from build123d import *

# Parameters (mm, degrees)
SKETCH1_W           = 151
SKETCH1_H           = 101.6
BOSS_EXTRUDE1_DEPTH = 3.8
SKETCH3_W           = 1.5
SKETCH3_H           = 3.5
CUT_EXTRUDE1_DEPTH  = 183.038457475
SKETCH4_W           = 10
SKETCH4_H           = 101.6
BOSS_EXTRUDE2_DEPTH = 3.8
SKETCH5_R           = 3
SKETCH5_R_2         = 1.75
CUT_EXTRUDE2_DEPTH  = 191.415335517
FILLET1_R           = 3
FILLET2_R           = 3
SKETCH6_W           = 3.8
SKETCH6_H           = 5.8
SKETCH6_H_2         = 10
SKETCH6_W_2         = 10
SKETCH6_H_3         = 3.8
SKETCH6_H_4         = 5
CUT_EXTRUDE3_DEPTH  = 191.415335517


with BuildPart() as part:
    # Sketch1 → Boss-Extrude1 (new body)
    with BuildSketch(Plane(origin=(0, 0, 0), x_dir=(1, 0, 0), z_dir=(0, 1, 0))):
        with Locations((75.5, -50.8)):
            Rectangle(SKETCH1_W, SKETCH1_H)
    extrude(amount=BOSS_EXTRUDE1_DEPTH)

    # Sketch3 → Cut-Extrude1 (cut, through all)
    with BuildSketch(Plane.XZ):
        with Locations((40.75, 87.6)):
            Rectangle(SKETCH3_W, SKETCH3_H)
        with Locations((48.25, 87.6)):
            Rectangle(SKETCH3_W, SKETCH3_H)
        with Locations((134.25, 87.6)):
            Rectangle(SKETCH3_W, SKETCH3_H)
        with Locations((141.75, 87.6)):
            Rectangle(SKETCH3_W, SKETCH3_H)
    extrude(amount=-CUT_EXTRUDE1_DEPTH, mode=Mode.SUBTRACT)

    # Sketch4 → Boss-Extrude2 (add, through all)
    with BuildSketch(Plane.XZ):
        with Locations((156, 50.8)):
            Rectangle(SKETCH4_W, SKETCH4_H)
    extrude(amount=-BOSS_EXTRUDE2_DEPTH)

    # Sketch5 → Cut-Extrude2 (cut, through all)
    with BuildSketch(Plane.XZ):
        with Locations(Location((155, 50.8, 0), (0, 0, 270))):
            Circle(SKETCH5_R)
        with Locations(Location((155, 91.6, 0), (0, 0, 270))):
            Circle(SKETCH5_R_2)
        with Locations(Location((155, 10, 0), (0, 0, 270))):
            Circle(SKETCH5_R_2)
    extrude(amount=-CUT_EXTRUDE2_DEPTH, mode=Mode.SUBTRACT)

    # Fillet1
    fillet1_edges = [part.edges().sort_by_distance(p)[0] for p in [
        (0, 1.9, 0),
        (0, 1.9, 101.6),
    ]]
    fillet(fillet1_edges, radius=FILLET1_R)

    # Fillet2
    fillet2_edges = [part.edges().sort_by_distance(p)[0] for p in [
        (161, 1.9, 101.6),
        (161, 1.9, 0),
    ]]
    fillet(fillet2_edges, radius=FILLET2_R)

    # Sketch6 → Cut-Extrude3 (cut, through all)
    with BuildSketch(Plane(origin=(0, 3.8, 0), x_dir=(1, 0, 0), z_dir=(0, 1, 0))):
        Polygon((148, -94), (148, -89.8), (144.2, -89.8), (144.2, -94.8), (138, -94.8), (138, -98.6), (148, -98.6), align=None)
        with Locations((146.1, -78.1)):
            Rectangle(SKETCH6_W, SKETCH6_H)
        with Locations((146.1, -51.8)):
            Rectangle(SKETCH6_W, SKETCH6_H_2)
        with Locations((146.1, -31.8)):
            Rectangle(SKETCH6_W, SKETCH6_H_2)
        with Locations((146.1, -11.8)):
            Rectangle(SKETCH6_W, SKETCH6_H_2)
        with Locations((135.5, -4.9)):
            Rectangle(SKETCH6_W_2, SKETCH6_H_3)
        with Locations((115.5, -4.9)):
            Rectangle(SKETCH6_W_2, SKETCH6_H_3)
        with Locations((95.5, -4.9)):
            Rectangle(SKETCH6_W_2, SKETCH6_H_3)
        with Locations((75.5, -4.9)):
            Rectangle(SKETCH6_W_2, SKETCH6_H_3)
        with Locations((55.5, -4.9)):
            Rectangle(SKETCH6_W_2, SKETCH6_H_3)
        with Locations((35.5, -4.9)):
            Rectangle(SKETCH6_W_2, SKETCH6_H_3)
        with Locations((15.5, -4.9)):
            Rectangle(SKETCH6_W_2, SKETCH6_H_3)
        with Locations((4.9, -11.8)):
            Rectangle(SKETCH6_W, SKETCH6_H_2)
        with Locations((4.9, -31.8)):
            Rectangle(SKETCH6_W, SKETCH6_H_2)
        with Locations((4.9, -51.8)):
            Rectangle(SKETCH6_W, SKETCH6_H_2)
        with Locations((4.9, -78.5)):
            Rectangle(SKETCH6_W, SKETCH6_H_4)
        Polygon((6.8, -94.8), (6.8, -89.8), (3, -89.8), (3, -94), (3, -98.6), (13, -98.6), (13, -94.8), align=None)
        with Locations((28, -96.7)):
            Rectangle(SKETCH6_W_2, SKETCH6_H_3)
        with Locations((48, -96.7)):
            Rectangle(SKETCH6_W_2, SKETCH6_H_3)
        with Locations((83, -96.7)):
            Rectangle(SKETCH6_W_2, SKETCH6_H_3)
        with Locations((103, -96.7)):
            Rectangle(SKETCH6_W_2, SKETCH6_H_3)
        with Locations((123, -96.7)):
            Rectangle(SKETCH6_W_2, SKETCH6_H_3)
    extrude(amount=-CUT_EXTRUDE3_DEPTH, mode=Mode.SUBTRACT)


solid = part.part
The model under review builds one solid part; all positions refer to its coordinate system, in mm. Coordinates: 2 decimals unless noted, no trailing zeros. Loops run counter-clockwise (first coordinate to the right, second up) from the corner with the lowest first, then second, coordinate; pieces in that order, holes last. Notation, with made-up numbers: M 42,5.25 L 80,5.25 A9 cw 80,20.25 Z; hole C 43.25,-31.75 d7. An arc over 180 degrees is marked long. Put each result on its own line as item: value. Start each with the question number.
Q1. Clearance check with a flat-ended pin moving along its axis: pin 1 (1 mm diameter, centred on x = 53.5, z = 83, fed in from -Y). State where the tip first meets the part, or that it passes through.
Q2. Add section B-B (z = 10). Write out the cut boundary in (x, y), and give its area (3 significant figures).
Q3. Add section A-A (x = 155). Write out the cut boundary in (y, z).
Q4. The part is to be moulded in two halves that separate along X. For faces 1 (the flat face through (110.5, 2, 5)), 2 (the cylindrical face through (0.9, 1.93, 0.86)), 3 (the flat face through (35, 2, 6.8)), 4 (the flat face through (79, 0, 52)), say which applies: +X half, -X half, draft (parallel to the pull), parting line (faces both ways), or undercut.
Q5. Wall thickness on line 1 (Z direction, x = 155, y = 1.5); line 2 (X direction, y = 1.8, z = 10); line 3 (X direction, y = 1.4, z = 79.5): over which ranges is each line inside the solid? List them lowest first.
Q6. Add section C-C (y = 1.2). Count the separate pieces of the cut face and the enclosed holes in it, and give its area (3 significant figures).
Answers:
1. pin 1: stops at y = 0
2. outline: M 0,0 L 3,0 L 3,3.8 L 0,3.8 Z; M 6.8,0 L 144.2,0 L 144.2,3.8 L 6.8,3.8 Z; M 148,0 L 153.25,0 L 153.25,3.8 L 148,3.8 Z; M 156.75,0 L 161,0 L 161,3.8 L 156.75,3.8 Z
2. area: 570 mm^2
3. outline: M 0,0 L 3.8,0 L 3.8,8.25 L 0,8.25 Z; M 0,11.75 L 3.8,11.75 L 3.8,47.8 L 0,47.8 Z; M 0,53.8 L 3.8,53.8 L 3.8,89.85 L 0,89.85 Z; M 0,93.35 L 3.8,93.35 L 3.8,101.6 L 0,101.6 Z
4. face 1: undercut
4. face 2: -X half
4. face 3: undercut
4. face 4: draft
5. line 1: z = 0 to 8.25, 11.75 to 47.8, 53.8 to 89.85, 93.35 to 101.6
5. line 2: x = 0 to 3, 6.8 to 144.2, 148 to 153.25, 156.75 to 161
5. line 3: x = 0 to 3, 6.8 to 144.2, 148 to 161
6. separate pieces: 1
6. enclosed holes: 29
6. area: 15,400 mm^2
